Autodesk Inventor part; units mm, degrees
ref_plane "YZ Plane" through (0, 0, 0) normal (1, 0, 0) x (0, 1, 0)
ref_plane "XZ Plane" through (0, 0, 0) normal (0, 1, 0) x (-1, 0, 0)
ref_plane "XY Plane" through (0, 0, 0) normal (0, 0, 1) x (1, 0, 0)
sketch "Sketch1" plane through (0, 0, 0) normal (0, 0, 1) x (1, 0, 0)
  line L0 (0, 0) -> (0, 1.5)
  line L1 (2.2, 3.8) -> (2.2, 2)
  line L2 (2.2, 2) -> (10.2, 2)
  line L3 (10.2, 2) -> (10.2, 0)
  line L4 (10.2, 0) -> (0, 0)
  line L5 (2.2, 3.8) -> (1.7, 3.8)
  arc A0 (1.7, 3.8) -> (0, 1.5) centre (4.0624, 0.2756) ccw
  dimension "d0" = 2.2
  dimension "d1" = 8
  dimension "d2" = 3.8
  dimension "d4" = 0.5
  dimension "d5" = 2
  dimension "d7" = 1.5
revolve "Revolution1" add sketch "Sketch1" angle 360 about axis through (10.2, 0, 0) along (-1, 0, 0)
sketch "Sketch2" plane through (0, 0, 0) normal (-1, 0, 0) x (0, 0, 1)
  line L0 (-1.25, -0.7217) -> (-1.25, 0.7217)
  line L1 (-1.25, 0.7217) -> (0, 1.4434)
  line L2 (0, 1.4434) -> (1.25, 0.7217)
  line L3 (1.25, 0.7217) -> (1.25, -0.7217)
  line L4 (1.25, -0.7217) -> (0, -1.4434)
  line L5 (0, -1.4434) -> (-1.25, -0.7217)
  point P0 (0, 0)
  point P1 (0, 0)
  dimension "d8" = 2.5
extrude "Extrusion1" cut sketch "Sketch2" against normal blind 1.3
chamfer "Chamfer1" distance 0.2 angle 45 1 edges at (10.2, -2, 0)
thread "Thread1"
properties part number "M4 x 8 mm BHCS"
Could you check a few things on this model? Use its own coordinates, in mm. A direction names the side the tool comes from. Give positions to 0.01 mm unless a question says otherwise; leave off trailing zeros. Order: outer loops, then holes, each group sorted by start corner. A loop starts at its lowest first (then second) coordinate and runs counter-clockwise, first axis right, second up.
Q1. For faces 1 (the flat face through (1.3, 0, 0)), 2 (the cylindrical face through (6, 0, -2)), which set-ups out of +Z, -Z, +X, -X, +Y, -Y let a thin tool reach every point of the face, with its end or its side?
Q2. I'm going to push flat-ended pins straight in: P1, Ø2, axis at x = 3, z = 2.5, coming from the +Y side; P2, Ø0.8, axis at y = 0.5, z = 0, coming from the -X side; P3, Ø4, axis at x = 2.5, y = 2.5, coming from the -Z side. Where does each tip first touch, or does it pass through?
Q3. Suppose I cut it at A-A, the plane x = 7.5. Write out the boundary of the cut face in (y, z), and give its area (3 significant figures).
Q4. If I drill on line 1 along Y through (x, z) = (0.5, -0.75); line 2 along Y through (x, z) = (1.75, -2.25); line 3 along Z through (x, y) = (8.5, -1.5), over which ranges is the centre line in solid material (lowest first)?
Q5. We'd pull the mould along Y, two halves only. Please class faces 3 (the flat face through (10.2, 0, 0)), 4 (the cylindrical face through (1.947, -3.796, -0.167)), 5 (the flat face through (1, 0, 1.25)): +Y half, -Y half, draft (parallel to the pull), parting line (faces both ways), or undercut.
Solution:
1. face 1: -X
1. face 2: +X
2. P1: stops at y = 3.29
2. P2: stops at x = 1.3
2. P3: stops at z = -3.76
3. outline: circle Ø4 at (0, 0)
3. area: 12.6 mm2
4. line 1: y = -2.47 to -1.01, 1.01 to 2.47
4. line 2: y = -3.06 to 3.06
4. line 3: z = -1.32 to 1.32
5. face 3: draft
5. face 4: parting line
5. face 5: undercut
